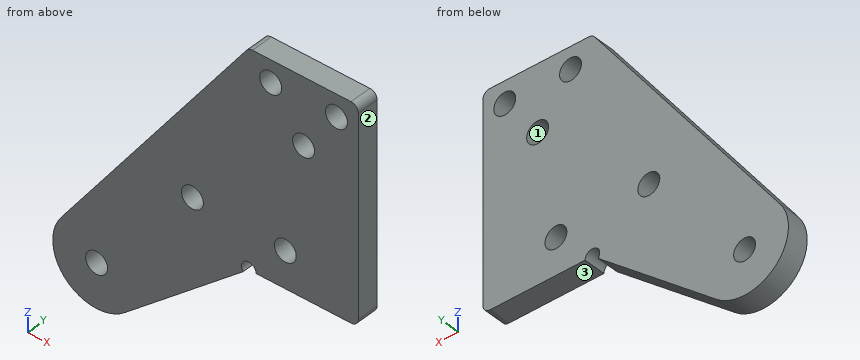
```python
from build123d import *

# Parameters (mm, degrees)
SKETCH_1_R          = 1.5
EXTRUDE_1_DEPTH     = 3
SKETCH_3_R          = 1
CUT_EXTRUDE_2_DEPTH = 131.490420233
FILLET_1_R          = 1


with BuildPart() as part:
    # 草图1 → 凸台-拉伸1 (new body)
    with BuildSketch(Plane(origin=(0, 0, 0), x_dir=(1, 0, 0), z_dir=(0, 1, 0))):
        with BuildLine():
            Line((-107.991031726, 54.61519926), (-91, 40.5))
            Line((-91, 40.5), (-76, 40.5))
            Line((-76, 40.5), (-76, 11.5))
            Line((-76, 11.5), (-91, 11.5))
            Line((-91, 11.5), (-116.661386977, 46.448923126))
            ThreePointArc((-116.661386977, 46.448923126), (-115.938856388, 54.367705823), (-107.991031726, 54.61519926))
        make_face()
        with Locations(Location((-111.825081255, 50, 0), (0, 0, 270))):
            Circle(SKETCH_1_R, mode=Mode.SUBTRACT)
        with Locations(Location((-88, 14.5, 0), (0, 0, 270))):
            Circle(SKETCH_1_R, mode=Mode.SUBTRACT)
        with Locations(Location((-79, 14.5, 0), (0, 0, 270))):
            Circle(SKETCH_1_R, mode=Mode.SUBTRACT)
        with Locations(Location((-83.5, 20.5, 0), (0, 0, 270))):
            Circle(SKETCH_1_R, mode=Mode.SUBTRACT)
        with Locations(Location((-86, 35.5, 0), (0, 0, 270))):
            Circle(SKETCH_1_R, mode=Mode.SUBTRACT)
        with Locations(Location((-98.71745767, 34.89403416, 0), (0, 0, 270))):
            Circle(SKETCH_1_R, mode=Mode.SUBTRACT)
    extrude(amount=EXTRUDE_1_DEPTH)

    # 草图3 → 切除-拉伸2 (cut, through all)
    with BuildSketch(Plane(origin=(0, 3, 0), x_dir=(1, 0, 0), z_dir=(0, 1, 0))):
        with Locations((-91, 40.5)):
            Circle(SKETCH_3_R)
    extrude(amount=-CUT_EXTRUDE_2_DEPTH, mode=Mode.SUBTRACT)

    # 圆角1
    fillet_1_edges = [part.edges().sort_by_distance(p)[0] for p in [
        (-76, 1.5, -40.5),
        (-76, 1.5, -11.5),
        (-91, 1.5, -11.5),
    ]]
    fillet(fillet_1_edges, radius=FILLET_1_R)


solid = part.part
```
Geometry check sheet. Reference: the model listing, model coordinates, mm. Face numbers are marked on the shaded views. Round coordinates to 2 decimals unless told otherwise and drop trailing zeros. Order: outer loops, then holes, each group sorted by start corner. A loop starts at its lowest first (then second) coordinate and runs counter-clockwise, first axis right, second up. Notation, with made-up numbers: (34.5, 40) - (57.5, 40) arc R15 cw to (57.5, 68) - close; hole circle Ø9 at (29.25, 56.5). An arc over 180 degrees is marked (long way). Use a Markdown table: item, result. Add a question column.
(1) Sectioned sample at B-B, the plane z = -50. Enter the section's corners in (x, y).
(2) Sectioned sample at C-C, the plane z = -14.5. Enter the section's corners in (x, y), and give its area (3 significant figures).
(3) Sectioned sample at A-A, the plane x = -79. Enter the section's corners in (y, z), and give its area (3 significant figures).
(4) Material ranges on line 1 along Z through (x, y) = (-87, 1.5); line 2 along Z through (x, y) = (-88, 1.45); line 3 along X through (y, z) = (1.5, -14.5), recorded low to high. Write a range as [from, to].
(5) Release check for a two-part mould opening along X. For the marked faces 1, 2 and 3 record: pulls with the +X half, pulls with the -X half, needs draft (parallel to the pull), parting line crosses it, or undercut.
(6) Sectioned sample at D-D, the plane y = 0.7. Enter the section's corners in (x, z), and give its area (3 significant figures).
Answers below:
| question | item | result |
|---|---|---|
| 1 | outline | (-117.83, 0) - (-113.33, 0) - (-113.33, 3) - (-117.83, 3) - close; (-110.33, 0) - (-102.44, 0) - (-102.44, 3) - (-110.33, 3) - close |
| 2 | outline | (-93.2, 0) - (-89.5, 0) - (-89.5, 3) - (-93.2, 3) - close; (-86.5, 0) - (-80.5, 0) - (-80.5, 3) - (-86.5, 3) - close; (-77.5, 0) - (-76, 0) - (-76, 3) - (-77.5, 3) - close |
| 2 | area | 33.6 mm² |
| 3 | outline | (0, -40.5) - (3, -40.5) - (3, -16) - (0, -16) - close; (0, -13) - (3, -13) - (3, -11.5) - (0, -11.5) - close |
| 3 | area | 78.0 mm² |
| 4 | line 1 | [-40.5, -36.62], [-34.38, -15.62], [-13.38, -11.5] |
| 4 | line 2 | [-40.5, -16], [-13, -11.5] |
| 4 | line 3 | [-93.2, -89.5], [-86.5, -80.5], [-77.5, -76] |
| 5 | face 1 | undercut |
| 5 | face 2 | pulls with the +X half |
| 5 | face 3 | needs draft |
| 6 | outline | (-116.66, -46.45) arc R6 ccw to (-107.99, -54.62) - (-91.77, -41.14) arc R1 cw (long way) to (-90, -40.5) - (-77, -40.5) arc R1 ccw to (-76, -39.5) - (-76, -12.5) arc R1 ccw to (-77, -11.5) - (-90.49, -11.5) arc R1 ccw to (-91.3, -11.91) - close; hole circle Ø3 at (-111.83, -50); hole circle Ø3 at (-98.72, -34.89); hole circle Ø3 at (-88, -14.5); hole circle Ø3 at (-86, -35.5); hole circle Ø3 at (-83.5, -20.5); hole circle Ø3 at (-79, -14.5) |
| 6 | area | 941 mm² |
